```python
from build123d import *

# Parameters (mm, degrees)
SKETCH1_R           = 10
SKETCH1_R_2         = 0.8
BOSS_EXTRUDE1_DEPTH = 8
FILLET1_R           = 2
CUT_EXTRUDE1_DEPTH  = 60


with BuildPart() as part:
    # Sketch1 → Boss-Extrude1 (new body)
    # profile 1 of 6: a face of its own
    with BuildSketch(Plane.XY):
        with BuildLine():
            ThreePointArc((10, 0), (0, -10), (-10, 0))
            Line((-10, 0), (-10, -80))
            ThreePointArc((-10, -80), (0, -70), (10, -80))
            Line((10, -80), (10, 0))
        make_face()
    # profile 2 of 6: a face of its own
    with BuildSketch(Plane.XY):
        Circle(SKETCH1_R)
        with Locations((-7, 0)):
            Circle(SKETCH1_R_2, mode=Mode.SUBTRACT)
        with Locations((0, -7)):
            Circle(SKETCH1_R_2, mode=Mode.SUBTRACT)
        with Locations((7, 0)):
            Circle(SKETCH1_R_2, mode=Mode.SUBTRACT)
        with Locations((0, 7)):
            Circle(SKETCH1_R_2, mode=Mode.SUBTRACT)
    # profile 3 of 6: a face of its own
    with BuildSketch(Plane.XY):
        with BuildLine():
            ThreePointArc((10, -80), (0, -70), (-10, -80))
            Line((-10, -80), (-2.1, -80))
            ThreePointArc((-2.1, -80), (0, -77.9), (2.1, -80))
            Line((2.1, -80), (10, -80))
        make_face()
    # profile 4 of 6: a face of its own
    with BuildSketch(Plane.XY):
        with BuildLine():
            Line((-2.1, -80), (-10, -80))
            ThreePointArc((-10, -80), (0, -90), (10, -80))
            Line((10, -80), (2.1, -80))
            ThreePointArc((2.1, -80), (0, -82.1), (-2.1, -80))
        make_face()
    # profile 5 of 6: a face of its own
    with BuildSketch(Plane.XY):
        with BuildLine():
            ThreePointArc((10, -80), (0, -70), (-10, -80))
            Line((-10, -80), (-2.1, -80))
            ThreePointArc((-2.1, -80), (0, -77.9), (2.1, -80))
            Line((2.1, -80), (10, -80))
        make_face()
    # profile 6 of 6: a face of its own
    with BuildSketch(Plane.XY):
        with BuildLine():
            Line((-2.1, -80), (-10, -80))
            ThreePointArc((-10, -80), (0, -90), (10, -80))
            Line((10, -80), (2.1, -80))
            ThreePointArc((2.1, -80), (0, -82.1), (-2.1, -80))
        make_face()
    extrude(amount=BOSS_EXTRUDE1_DEPTH)

    # Fillet1
    fillet1_edges = [part.edges().sort_by_distance(p)[0] for p in [
        (-10, -40, 0),
        (0, 10, 0),
        (10, -40, 0),
        (0, -90, 0),
    ]]
    fillet(fillet1_edges, radius=FILLET1_R)

    # Sketch3 → Cut-Extrude1 (cut)
    with BuildSketch(Plane(origin=(0, 0, 0), x_dir=(-1, 0, 0), z_dir=(0, 0, -1))):
        with BuildLine():
            Line((-5, -65), (-5, -15))
            ThreePointArc((-5, -15), (0, -10), (5, -15))
            Line((5, -15), (5, -65))
            ThreePointArc((5, -65), (0, -70), (-5, -65))
        make_face()
    extrude(amount=-CUT_EXTRUDE1_DEPTH, mode=Mode.SUBTRACT)


solid = part.part
```
Check sheet for the modelled part. Datum: model origin and axes. Units: mm. A direction names the side the tool comes from. Coordinates: 2 decimals unless noted, no trailing zeros. Write each loop counter-clockwise with the first axis right and the second up, starting at its lowest first coordinate (ties: lowest second). Pieces come first, ordered by that corner, then holes. Notation, with made-up numbers: (11.5, 33) - (24.5, 33) arc R23 ccw to (24.5, 54) - close; hole circle Ø6 at (64.5, 25). An arc over 180 degrees is marked (long way). One line per question, with ' | ' between items.
Item 1: Access from +Z, -Z, +X, -X, +Y, -Y to the whole of each face (thin tool, end or side, straight path). Record for faces 4 (the face through (-10, -39, 5)), 5 (the face through (0, -70, 4)).
Determined:
face 4: +Z, -Z, -X, +Y, -Y | face 5: +Z, -Z
Item 2: Sectioned sample at A-A on y = -56. Record the boundary of the cut face in (x, z).
Determined:
outline: (-10, 2) arc R2 ccw to (-8, 0) - (-5, 0) - (-5, 8) - (-10, 8) - close; (5, 0) - (8, 0) arc R2 ccw to (10, 2) - (10, 8) - (5, 8) - close
Item 3: Thickness scan on line 1 (Y direction, x = 0, z = 4.25); line 2 (X direction, y = -41.5, z = 2); line 3 (X direction, y = -80, z = 2). Record the ranges inside material, lowest first. Write a range as [from, to].
Determined:
line 1: y = [-90, -82.1], [-77.9, -70], [-10, -7.8], [-6.2, 6.2], [7.8, 10] | line 2: x = [-10, -5], [5, 10] | line 3: x = [-10, -2.1], [2.1, 10]
Item 4: Sectioned sample at B-B on z = 6.75. Record the boundary of the cut face in (x, y).
Determined:
outline: (-10, -80) arc R10 ccw to (10, -80) - (10, 0) arc R10 ccw to (-10, 0) - close; hole circle Ø1.6 at (-7, 0); hole (-5, -65) arc R5 ccw to (5, -65) - (5, -15) arc R5 ccw to (-5, -15) - close; hole circle Ø4.2 at (0, -80); hole circle Ø1.6 at (0, -7); hole circle Ø1.6 at (0, 7); hole circle Ø1.6 at (7, 0)
Item 5: Mould release check, pull along Y, two halves, no side actions. Record for faces 1 (the face through (6.2, 0, 3.9)), 2 (the face through (0, 10, 5)), 3 (the face through (10, -41, 5)): pulls with the +Y half, pulls with the -Y half, needs draft (parallel to the pull), parting line crosses it, or undercut.
Determined:
face 1: undercut | face 2: pulls with the +Y half | face 3: needs draft
Item 6: Gauge pin test, flat end, axial feed: P1, Ø2.5, axis at x = -7, y = 0, coming from the -Z side. Record the tip position at first contact, or that the pin passes through.
Determined:
P1: stops at z = 0
